For this review, take the finished solid that the model builds, in its own axes (mm). A direction names the side the tool comes from. Give positions to 0.01 mm unless a question says otherwise; leave off trailing zeros. Order: outer loops, then holes, each group sorted by start corner. A loop starts at its lowest first (then second) coordinate and runs counter-clockwise, first axis right, second up.
Item 1: Consider section B-B (y = 30.5). Give the boundary of the cut face in (x, z).
Item 2: Consider section D-D (y = 8). Give the boundary of the cut face in (x, z), plus the area to 3 significant figures.
Item 3: The part is to be moulded in two halves that separate along X. For faces 1 (the cylindrical face through (44, 5, 6)), 2 (the flat face through (6, 10, 6)), 3 (the flat face through (26, 0, 20)), 4 (the flat face through (52, 13, 20)), say which applies: released by +X, released by -X, zero draft, split by the parting line, or undercut.
Item 4: For probe 1 along X at (y, z) = (3.5, 6); probe 2 along Y at (x, z) = (26, 30.5); probe 3 along X at (y, z) = (11.5, 9.5), list the stretches that pass through material, from the lowest coordinate up.
Item 5: For P1, Ø3, axis at x = 45, z = 33.5, coming from the -Y side; P2, Ø2, axis at x = 27.5, y = 30, coming from the -Z side; P3, Ø5, axis at x = 46, z = 6, coming from the +Y side; P4, Ø1.2, axis at x = 45.5, z = 6.5, coming from the -Y side, all flat-tipped, find the tip position at first contact; note any pin that passes through.
Item 6: Consider section C-C (z = 33). Give the boundary of the cut face in (x, y), plus the area to 3 significant figures.
Item 7: Machinability: for faces 5 (the flat face through (46, 10, 6)), 6 (the flat face through (26, 37.738, 20)), which of the approach directions +Z, -Z, +X, -X, +Y, -Y give a long, thin tool a straight path to every point of the face, cutting with its end or side? Answer none if there is none.
Item 8: Consider section A-A (x = 32). Give the boundary of the cut face in (y, z), plus the area to 3 significant figures.
```python
from build123d import *

# Parameters (mm, degrees)
SKETCH1_R           = 14
BOSS_EXTRUDE1_DEPTH = 40
SKETCH2_R           = 2
CUT_EXTRUDE1_DEPTH  = 10


with BuildPart() as part:
    # Sketch1 → Boss-Extrude1 (new body)
    with BuildSketch(Plane.XY):
        Polygon((0, 0), (52, 0), (52, 27), (40, 37.737759826), (12, 37.737759826), (0, 27), align=None)
        with Locations((26, 18.157759826)):
            Circle(SKETCH1_R, mode=Mode.SUBTRACT)
    extrude(amount=BOSS_EXTRUDE1_DEPTH)

    # Sketch2 → Cut-Extrude1 (cut)
    with BuildSketch(Plane.XZ):
        with Locations(Location((6, 34, 0), (0, 0, 270))):
            Circle(SKETCH2_R)
        with Locations(Location((46, 34, 0), (0, 0, 270))):
            Circle(SKETCH2_R)
        with Locations(Location((6, 6, 0), (0, 0, 270))):
            Circle(SKETCH2_R)
        with Locations(Location((46, 6, 0), (0, 0, 270))):
            Circle(SKETCH2_R)
    extrude(amount=-CUT_EXTRUDE1_DEPTH, mode=Mode.SUBTRACT)


solid = part.part
```
Resolved:
1. outline: (3.91, 0) - (19.39, 0) - (19.39, 40) - (3.91, 40) - close; (32.61, 0) - (48.09, 0) - (48.09, 40) - (32.61, 40) - close
2. outline: (0, 0) - (16.37, 0) - (16.37, 40) - (0, 40) - close; (35.63, 0) - (52, 0) - (52, 40) - (35.63, 40) - close; hole circle Ø4 at (6, 6); hole circle Ø4 at (6, 34); hole circle Ø4 at (46, 6); hole circle Ø4 at (46, 34)
2. area: 1,260 mm2
3. face 1: undercut
3. face 2: undercut
3. face 3: zero draft
3. face 4: released by +X
4. probe 1: x = 0 to 4, 8 to 44, 48 to 52
4. probe 2: y = 0 to 4.16, 32.16 to 37.74
4. probe 3: x = 0 to 13.68, 38.32 to 52
5. P1: stops at y = 0
5. P2: passes through
5. P3: stops at y = 34.61
5. P4: stops at y = 10
6. outline: (0, 0) - (4.27, 0) - (4.27, 10) - (7.73, 10) - (7.73, 0) - (44.27, 0) - (44.27, 10) - (47.73, 10) - (47.73, 0) - (52, 0) - (52, 27) - (40, 37.74) - (12, 37.74) - (0, 27) - close; hole circle Ø28 at (26, 18.16)
6. area: 1,150 mm2
7. face 5: -Y
7. face 6: +Z, -Z, +X, -X, +Y
8. outline: (0, 0) - (5.51, 0) - (5.51, 40) - (0, 40) - close; (30.81, 0) - (37.74, 0) - (37.74, 40) - (30.81, 40) - close
8. area: 498 mm2
